```python
from build123d import *

# Parameters (mm, degrees)
BOSS_EXTRUDE1_START = -34.9
SKETCH1_W           = 43.6
SKETCH1_H           = 18.5
BOSS_EXTRUDE1_DEPTH = 2.1
CUT_EXTRUDE1_START  = -34.9
SKETCH2_R           = 3.55
CUT_EXTRUDE1_DEPTH  = 2.1
CUT_EXTRUDE2_START  = -34.9
CUT_EXTRUDE2_DEPTH  = 2.1
BOSS_EXTRUDE2_START = 14.1
SKETCH4_R           = 6.5
BOSS_EXTRUDE2_DEPTH = 2.1
BOSS_EXTRUDE3_START = 14.1
SKETCH5_W           = 20.8
SKETCH5_H           = 13
BOSS_EXTRUDE3_DEPTH = 2.1
CUT_EXTRUDE3_START  = 14.1
SKETCH6_R           = 3.55
CUT_EXTRUDE3_DEPTH  = 2.1
CUT_EXTRUDE4_START  = 14.1
CUT_EXTRUDE4_DEPTH  = 2.1
BOSS_EXTRUDE4_START = -24.5
SKETCH8_R           = 6.5
BOSS_EXTRUDE4_DEPTH = 1.5
BOSS_EXTRUDE5_START = -24.5
SKETCH9_W           = 20.8
SKETCH9_H           = 13
BOSS_EXTRUDE5_DEPTH = 1.5
CUT_EXTRUDE5_START  = -24.5
SKETCH10_R          = 2.95
CUT_EXTRUDE5_DEPTH  = 1.5
BOSS_EXTRUDE6_START = -25.7
SKETCH11_W          = 42.2
SKETCH11_H          = 18.5
BOSS_EXTRUDE6_DEPTH = 1.7
BOSS_EXTRUDE7_START = -73.5
SKETCH12_R          = 6.5
BOSS_EXTRUDE7_DEPTH = 1.5
BOSS_EXTRUDE8_START = -73.5
SKETCH13_W          = 27.4
SKETCH13_H          = 18.5
BOSS_EXTRUDE8_DEPTH = 1.5
CUT_EXTRUDE6_START  = -73.5
SKETCH14_R          = 2.95
CUT_EXTRUDE6_DEPTH  = 1.5


with BuildPart() as part:
    # Sketch1 → Boss-Extrude1 (new, symmetric)
    with BuildSketch(Plane(origin=(0, 0, 0), x_dir=(0, 0, -1), z_dir=(1, 0, 0)).offset(BOSS_EXTRUDE1_START)):
        with Locations((5.6, 21.25)):
            Rectangle(SKETCH1_W, SKETCH1_H)
    extrude(amount=BOSS_EXTRUDE1_DEPTH, both=True)

    # Sketch2 → Cut-Extrude1 (cut, symmetric)
    with BuildSketch(Plane(origin=(0, 0, 0), x_dir=(0, 0, -1), z_dir=(1, 0, 0)).offset(CUT_EXTRUDE1_START)):
        with Locations((0, 24)):
            Circle(SKETCH2_R)
    extrude(amount=CUT_EXTRUDE1_DEPTH, both=True, mode=Mode.SUBTRACT)

    # Sketch3 → Cut-Extrude2 (cut, symmetric)
    with BuildSketch(Plane(origin=(0, 0, 0), x_dir=(0, 0, -1), z_dir=(1, 0, 0)).offset(CUT_EXTRUDE2_START)):
        Polygon((0, 20.45), (12.7, 21.596718595), (12.7, 26.403281405), (0, 27.55), align=None)
    extrude(amount=CUT_EXTRUDE2_DEPTH, both=True, mode=Mode.SUBTRACT)



with BuildPart() as body_2:
    # Sketch4 → Boss-Extrude2 (new, symmetric)
    with BuildSketch(Plane.XY.offset(BOSS_EXTRUDE2_START)):
        with Locations((-16.2, 18.5)):
            Circle(SKETCH4_R)
    extrude(amount=BOSS_EXTRUDE2_DEPTH, both=True)


with BuildPart() as part_1:
    add(part.part)

    add(body_2.part)  # Boss-Extrude3 merges body 2
    # Sketch5 → Boss-Extrude3 (add, symmetric)
    with BuildSketch(Plane.XY.offset(BOSS_EXTRUDE3_START)):
        with Locations((-26.6, 18.5)):
            Rectangle(SKETCH5_W, SKETCH5_H)
    extrude(amount=BOSS_EXTRUDE3_DEPTH, both=True)

    # Sketch6 → Cut-Extrude3 (cut, symmetric)
    with BuildSketch(Plane.XY.offset(CUT_EXTRUDE3_START)):
        with Locations((-16.2, 18.5)):
            Circle(SKETCH6_R)
    extrude(amount=CUT_EXTRUDE3_DEPTH, both=True, mode=Mode.SUBTRACT)

    # Sketch7 → Cut-Extrude4 (cut, symmetric)
    with BuildSketch(Plane.XY.offset(CUT_EXTRUDE4_START)):
        Polygon((-16.2, 22.103784861), (-28.9, 20.903281405), (-28.9, 16.096718595), (-16.2, 14.95), align=None)
    extrude(amount=CUT_EXTRUDE4_DEPTH, both=True, mode=Mode.SUBTRACT)



with BuildPart() as body_2_2:
    # Sketch8 → Boss-Extrude4 (new, symmetric)
    with BuildSketch(Plane.XY.offset(BOSS_EXTRUDE4_START)):
        with Locations(Location((-16.2, 18.5, 0), (0, 0, 180))):
            Circle(SKETCH8_R)
    extrude(amount=BOSS_EXTRUDE4_DEPTH, both=True)


with BuildPart() as part_2:
    add(part_1.part)

    add(body_2_2.part)  # Boss-Extrude5 merges body 2 2
    # Sketch9 → Boss-Extrude5 (add, symmetric)
    with BuildSketch(Plane.XY.offset(BOSS_EXTRUDE5_START)):
        with Locations((-26.6, 18.5)):
            Rectangle(SKETCH9_W, SKETCH9_H)
    extrude(amount=BOSS_EXTRUDE5_DEPTH, both=True)

    # Sketch10 → Cut-Extrude5 (cut, symmetric)
    with BuildSketch(Plane.XY.offset(CUT_EXTRUDE5_START)):
        with Locations((-16.2, 18.5)):
            Circle(SKETCH10_R)
    extrude(amount=CUT_EXTRUDE5_DEPTH, both=True, mode=Mode.SUBTRACT)

    # Sketch11 → Boss-Extrude6 (add, symmetric)
    with BuildSketch(Plane.XY.offset(BOSS_EXTRUDE6_START)):
        with Locations((-53.9, 21.25)):
            Rectangle(SKETCH11_W, SKETCH11_H)
    extrude(amount=BOSS_EXTRUDE6_DEPTH, both=True)



with BuildPart() as body_2_3:
    # Sketch12 → Boss-Extrude7 (new, symmetric)
    with BuildSketch(Plane(origin=(0, 0, 0), x_dir=(0, 0, -1), z_dir=(1, 0, 0)).offset(BOSS_EXTRUDE7_START)):
        with Locations((0, 24)):
            Circle(SKETCH12_R)
    extrude(amount=BOSS_EXTRUDE7_DEPTH, both=True)


with BuildPart() as part_3:
    add(part_2.part)

    add(body_2_3.part)  # Boss-Extrude8 merges body 2 3
    # Sketch13 → Boss-Extrude8 (add, symmetric)
    with BuildSketch(Plane(origin=(0, 0, 0), x_dir=(0, 0, -1), z_dir=(1, 0, 0)).offset(BOSS_EXTRUDE8_START)):
        with Locations((13.7, 21.25)):
            Rectangle(SKETCH13_W, SKETCH13_H)
    extrude(amount=BOSS_EXTRUDE8_DEPTH, both=True)

    # Sketch14 → Cut-Extrude6 (cut, symmetric)
    with BuildSketch(Plane(origin=(0, 0, 0), x_dir=(0, 0, -1), z_dir=(1, 0, 0)).offset(CUT_EXTRUDE6_START)):
        with Locations((0, 24)):
            Circle(SKETCH14_R)
    extrude(amount=CUT_EXTRUDE6_DEPTH, both=True, mode=Mode.SUBTRACT)


solid = part_3.part
```
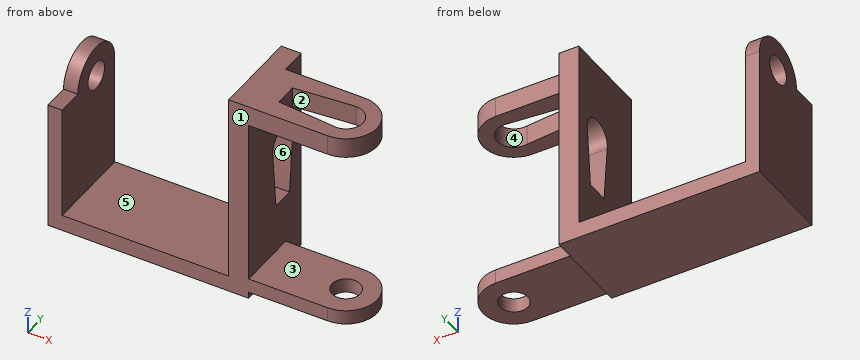
Input: part model. Units: mm. Frame: model coordinates. Face numbers are marked on the shaded views. A direction names the side the tool comes from. Coordinates: 2 decimals unless noted, no trailing zeros. Loops run counter-clockwise (first coordinate to the right, second up) from the corner with the lowest first, then second, coordinate; pieces in that order, holes last. Notation, with made-up numbers: (75.25, 50.5) -> (85.25, 50.5) arc R8 ccw to (85.25, 59.5) -> close; hole circle Ø2 at (87.25, 15). An arc over 180 degrees is marked (long way). Use a Markdown table: item, result.
1) Material intervals for line 1 along X through (y, z) = (18.5, 13); line 2 along Y through (x, z) = (-35, 0); line 3 along Y through (x, z) = (-16.2, -23.6), sorted ascending. Write a range as from..to.
Results found:
| item | result |
|---|---|
| line 1 | x = -37..-28.9, -12.65..-9.7 |
| line 2 | y = 12..20.45, 27.55..30.5 |
| line 3 | y = 12..15.55, 21.45..25 |
2) Cut plane A-A (x = -30.5). Return the cut outline in (y, z), then the cut area to 3 significant figures.
Results found:
| item | result |
|---|---|
| outline | (12, -26) -> (25, -26) -> (25, -23) -> (12, -23) -> close; (12, 12) -> (25, 12) -> (25, 16.2) -> (12, 16.2) -> close |
| area | 93.6 mm2 |
3) Cut plane D-D (y = 24). Return the cut outline in (x, z), then the cut area to 3 significant figures.
Results found:
| item | result |
|---|---|
| outline | (-75, -27.4) -> (-32.8, -27.4) -> (-32.8, -26) -> (-12.74, -26) -> (-12.74, -23) -> (-32.8, -23) -> (-32.8, -12.7) -> (-37, -12.7) -> (-37, -24) -> (-72, -24) -> (-72, -2.95) -> (-75, -2.95) -> close; (-75, 2.95) -> (-72, 2.95) -> (-72, 6.5) -> (-75, 6.5) -> close; (-37, 3.55) -> (-32.8, 3.55) -> (-32.8, 12) -> (-12.74, 12) -> (-12.74, 16.2) -> (-37, 16.2) -> close |
| area | 462 mm2 |
4) Cut plane B-B (z = -16). Return the cut outline in (x, y), then the cut area to 3 significant figures.
Results found:
| item | result |
|---|---|
| outline | (-75, 12) -> (-72, 12) -> (-72, 30.5) -> (-75, 30.5) -> close; (-37, 12) -> (-32.8, 12) -> (-32.8, 30.5) -> (-37, 30.5) -> close |
| area | 133 mm2 |
5) Contact query for flat-ended pins moving along their axis: pin 1 (4 mm diameter, centred on x = -20.5, y = 16, fed in from -Z); pin 2 (9 mm diameter, centred on y = 20, z = 1.5, fed in from +X); pin 3 (2 mm diameter, centred on x = -21.5, z = 14, fed in from +Y). Output: stop coordinate, or through.
Results found:
| item | result |
|---|---|
| pin 1 | stops at z = -26 |
| pin 2 | stops at x = -32.8 |
| pin 3 | stops at y = 25 |
6) Cut plane C-C (x = -23). Return the cut outline in (y, z), then the cut area to 3 significant figures.
Results found:
| item | result |
|---|---|
| outline | (12, -26) -> (25, -26) -> (25, -23) -> (12, -23) -> close; (12, 12) -> (15.56, 12) -> (15.56, 16.2) -> (12, 16.2) -> close; (21.46, 12) -> (25, 12) -> (25, 16.2) -> (21.46, 16.2) -> close |
| area | 68.8 mm2 |
7) Pull-direction query (Y, two-part tool) for the marked faces 1, 2 and 3; classes: released by +Y, released by -Y, zero draft, split by the parting line, or undercut.
Results found:
| item | result |
|---|---|
| face 1 | released by -Y |
| face 2 | undercut |
| face 3 | zero draft |
8) Access query for the marked faces 4, 5 and 6. Directions: +Z, -Z, +X, -X, +Y, -Y. A direction counts if a zero-diameter tool reaches every point of the face in a straight line with its end or side. Return the directions, or none.
Results found:
| item | result |
|---|---|
| face 4 | +Z |
| face 5 | +Z, +Y, -Y |
| face 6 | +X |
